Check sheet for the drawn part. Datum: minimum x, y, z corner. Units: mm. Coordinates: 2 decimals unless noted, no trailing zeros. Loops run counter-clockwise (first coordinate to the right, second up) from the corner with the lowest first, then second, coordinate; pieces in that order, holes last.
Q1. Go/stop test with a flat-tipped pin: P1, Ø2, axis at x = 7, y = 2.5, coming from the +Z side. Record where the tip stops, or that it passes through.
Q2. Material ranges on probe 1 along Y at (x, z) = (10, 0.15); probe 2 along X at (y, z) = (6.25, 0.3) (1 decimal); probe 3 along X at (y, z) = (9, 0.8) (1 decimal), recorded low to high.
Q3. Sectioned sample at B-B (x = 3.5). Enter the section's corners in (y, z) (1 decimal).
Q4. Mould release check, pull along Y, two halves, no side actions. Record for the marked faces 1, 2 and 3: +Y half, -Y half, draft (parallel to the pull), parting line (faces both ways), or undercut.
Q5. Sectioned sample at C-C (y = 9.25). Enter the section's corners in (x, z) (1 decimal).
Q6. Sectioned sample at A-A (z = 1.1). Enter the section's corners in (x, y) (1 decimal).
Q7. Sectioned sample at D-D (x = 15.75). Enter the section's corners in (y, z).
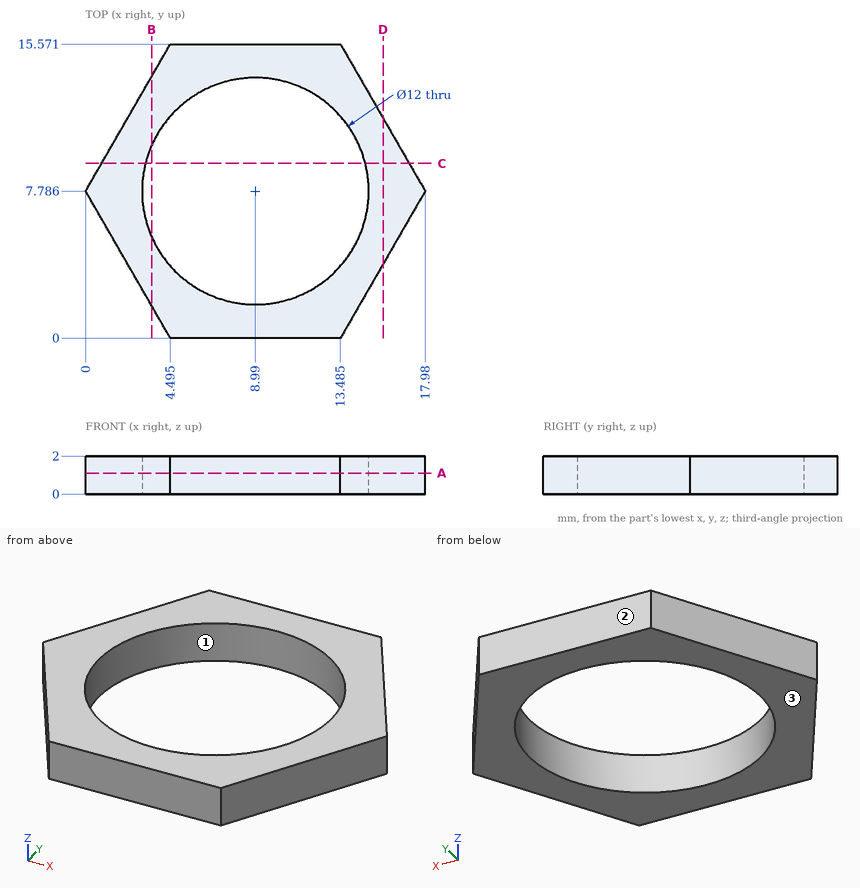
Geometry check:
1. P1: stops at z = 2
2. probe 1: y = 0 to 1.87, 13.7 to 15.57
2. probe 2: x = 0.9 to 3.2, 14.8 to 17.1
2. probe 3: x = 0.7 to 3.1, 14.9 to 17.3
3. outline: (1.7, 0) - (5.4, 0) - (5.4, 2) - (1.7, 2) - close; (10.2, 0) - (13.8, 0) - (13.8, 2) - (10.2, 2) - close
4. face 1: undercut
4. face 2: +Y half
4. face 3: draft
5. outline: (0.8, 0) - (3.2, 0) - (3.2, 2) - (0.8, 2) - close; (14.8, 0) - (17.1, 0) - (17.1, 2) - (14.8, 2) - close
6. outline: (0, 7.8) - (4.5, 0) - (13.5, 0) - (18, 7.8) - (13.5, 15.6) - (4.5, 15.6) - close; hole circle Ø12 at (9, 7.8)
7. outline: (3.92, 0) - (11.65, 0) - (11.65, 2) - (3.92, 2) - close
